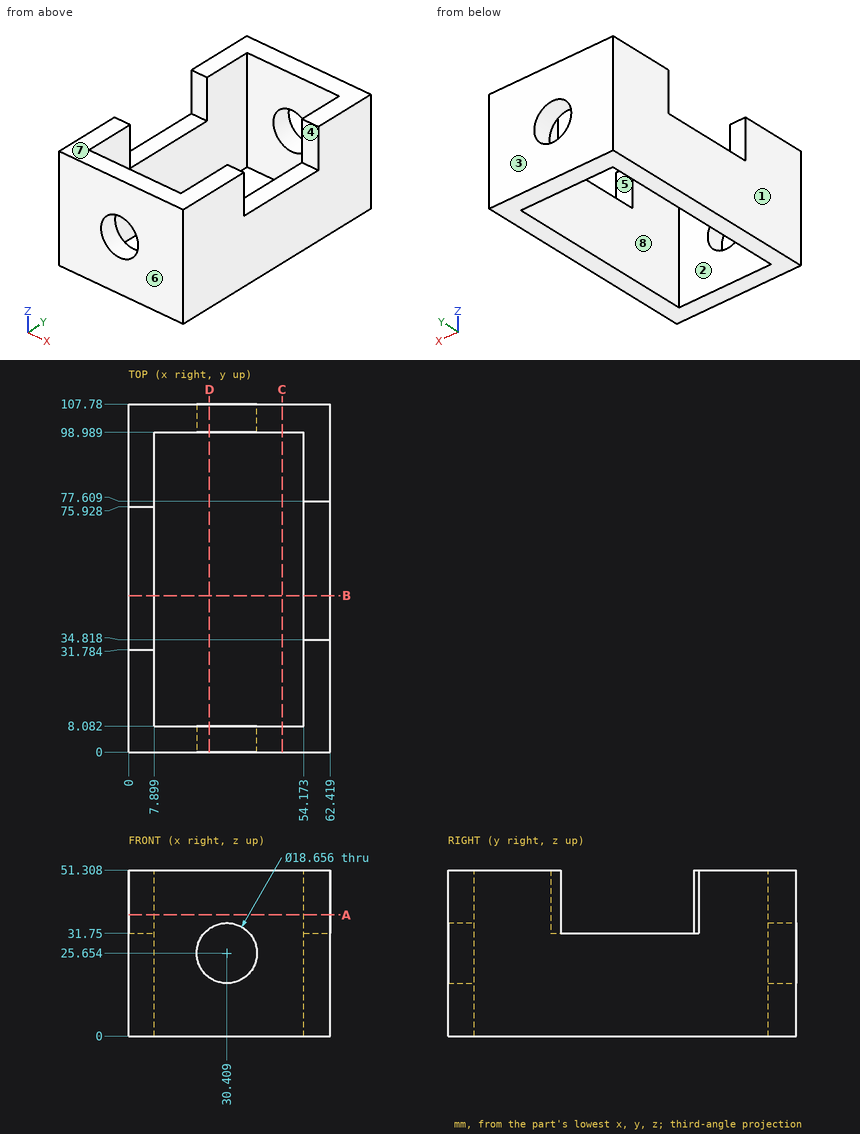
The drawing under review shows one solid part. Ordinate dimensions are in mm from its lowest x, y, z. A direction names the side the tool comes from. Coordinates: 2 decimals unless noted, no trailing zeros. Write each loop counter-clockwise with the first axis right and the second up, starting at its lowest first coordinate (ties: lowest second). Pieces come first, ordered by that corner, then holes. Notation, with made-up numbers: (3, -9) - (46, -9) arc R22 ccw to (46, 27) - close; hole circle Ø6 at (39.25, 8.25). An arc over 180 degrees is marked (long way). Use one line per item in the form item = value.
Q1. Consider section A-A (z = 37.5). Write out the cut boundary in (x, y).
Taken from the geometry:
outline = (0, 0) - (62.42, 0) - (62.42, 34.82) - (54.17, 34.82) - (54.17, 8.08) - (7.9, 8.08) - (7.9, 31.78) - (0, 31.78) - close; (0, 75.93) - (7.9, 75.93) - (7.9, 98.99) - (54.17, 98.99) - (54.17, 77.61) - (62.42, 77.61) - (62.42, 107.78) - (0, 107.78) - close
Q2. The part is to be moulded in two halves that separate along Y. For the marked faces 6, 7 and 8, say which applies: +Y half, -Y half, draft (parallel to the pull), parting line (faces both ways), or undercut.
Taken from the geometry:
face_6 = -Y half
face_7 = draft
face_8 = undercut
Q3. Consider section C-C (x = 47.5). Write out the cut boundary in (y, z), plus the area to 3 significant figures.
Taken from the geometry:
outline = (0, 0) - (8.08, 0) - (8.08, 51.31) - (0, 51.31) - close; (98.99, 0) - (107.78, 0) - (107.78, 51.31) - (98.99, 51.31) - close
area = 866 mm^2
Q4. Insertion check: pin 1 Ø6.5 at (x, y) = (3, 54.5) entering from +Z. The pin has a flat end and moves straight along its axis. Give the tip position at first contact, or say it passes through.
Taken from the geometry:
pin_1 = 31.75
Q5. Consider section D-D (x = 25). Write out the cut boundary in (y, z) (1 decimal).
Taken from the geometry:
outline = (0, 0) - (8.1, 0) - (8.1, 18.1) - (0, 18.1) - close; (0, 33.3) - (8.1, 33.3) - (8.1, 51.3) - (0, 51.3) - close; (99, 0) - (107.8, 0) - (107.8, 18.1) - (99, 18.1) - close; (99, 33.3) - (107.8, 33.3) - (107.8, 51.3) - (99, 51.3) - close
Q6. Machinability: for the marked faces 1, 2, 3, 4 and 5, which of the approach directions +Z, -Z, +X, -X, +Y, -Y give a long, thin tool a straight path to every point of the face, cutting with its end or side? Answer none if there is none.
Taken from the geometry:
face_1 = +Z, -Z, -X, +Y, -Y
face_2 = +Z, -Z
face_3 = +Z, -Z, +X, -X, +Y
face_4 = +Z, +X
face_5 = +Z, +X, -X
Q7. For probe 1 along Y at (x, z) = (35.5, 2); probe 2 along X at (y, z) = (93, 30.5); probe 3 along Z at (x, y) = (3.5, 64.5), list the stretches that pass through material, from the lowest coordinate up.
Taken from the geometry:
probe_1 = 0 to 8.08, 98.99 to 107.78
probe_2 = 0 to 7.9, 54.17 to 62.42
probe_3 = 0 to 31.75
Q8. Consider section B-B (y = 48.5). Write out the cut boundary in (x, z).
Taken from the geometry:
outline = (0, 0) - (7.9, 0) - (7.9, 31.75) - (0, 31.75) - close; (54.17, 0) - (62.42, 0) - (62.42, 31.75) - (54.17, 31.75) - close
